Verification items for this drawing (mm, ordinates from the low corner). A direction names the side the tool comes from. Round coordinates to 2 decimals unless told otherwise and drop trailing zeros. Order: outer loops, then holes, each group sorted by start corner. A loop starts at its lowest first (then second) coordinate and runs counter-clockwise, first axis right, second up. Notation, with made-up numbers: (73.5, 54.5) -> (129.5, 54.5) arc R31 ccw to (129.5, 84.5) -> close; hole circle Ø1 at (-22.5, -27.75). An arc over 180 degrees is marked (long way). Put each result on its own line as item: value.
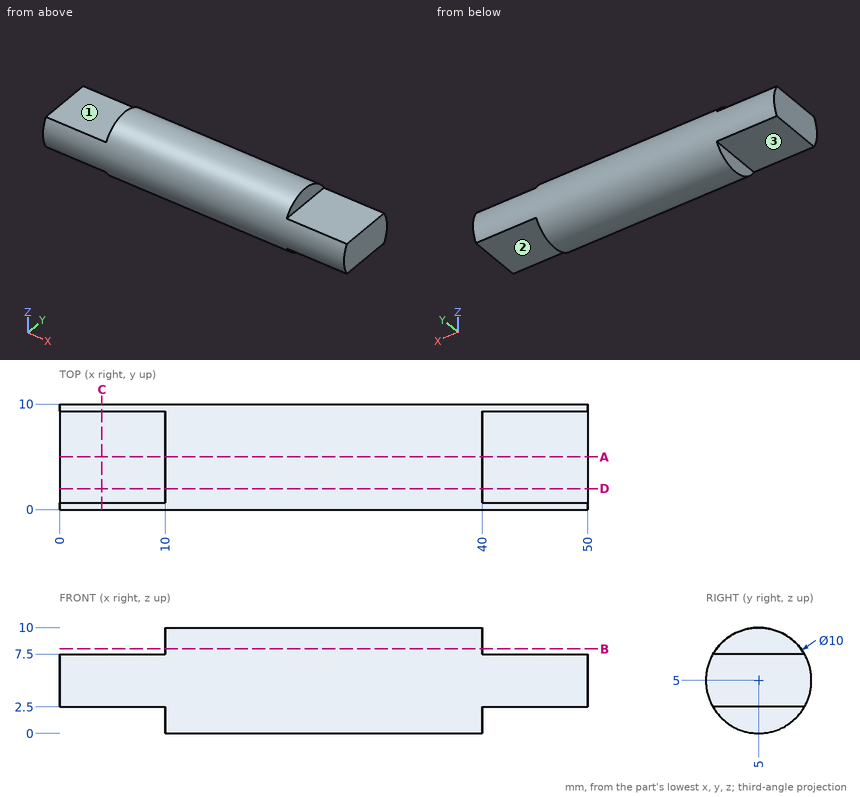
Item 1: Section check B-B on z = 8. Record the boundary of the cut face in (x, y), then the cut area to 3 significant figures.
Check sheet entries:
outline: (10, 1) -> (40, 1) -> (40, 9) -> (10, 9) -> close
area: 240 mm^2
Item 2: Material ranges on L1, parallel to X at y = 1.5, z = 8.5; L2, parallel to Z at x = 6, y = 6.5; L3, parallel to Z at x = 19, y = 4.75, recorded low to high. Write a range as [from, to].
Check sheet entries:
L1: x = [10, 40]
L2: z = [2.5, 7.5]
L3: z = [0.01, 9.99]
Item 3: Section check D-D on y = 2. Record the boundary of the cut face in (x, z), then the cut area to 3 significant figures.
Check sheet entries:
outline: (0, 2.5) -> (10, 2.5) -> (10, 1) -> (40, 1) -> (40, 2.5) -> (50, 2.5) -> (50, 7.5) -> (40, 7.5) -> (40, 9) -> (10, 9) -> (10, 7.5) -> (0, 7.5) -> close
area: 340 mm^2
Item 4: Tool access check on the marked faces 1, 2 and 3. Record the directions out of +Z, -Z, +X, -X, +Y, -Y that give a thin tool (end or side, any length) a straight path to the whole face; none if there is none.
Check sheet entries:
face 1: +Z, -X, +Y, -Y
face 2: -Z, +X, +Y, -Y
face 3: -Z, -X, +Y, -Y
Item 5: Gauge pin test, flat ends, axial feed: pin 1 Ø4 at (x, y) = (35.5, 3.5) entering from +Z; pin 2 Ø1.2 at (y, z) = (6.5, 8.5) entering from -X; pin 3 Ø0.8 at (y, z) = (6.5, 1.5) entering from +X; pin 4 Ø4.5 at (x, y) = (3.5, 4) entering from -Z. Record the tip position at first contact, or that the pin passes through.
Check sheet entries:
pin 1: stops at z = 10
pin 2: stops at x = 10
pin 3: stops at x = 40
pin 4: stops at z = 2.5
Item 6: Section check C-C on x = 4. Record the boundary of the cut face in (y, z).
Check sheet entries:
outline: (0.67, 2.5) -> (9.33, 2.5) arc R5 ccw to (9.33, 7.5) -> (0.67, 7.5) arc R5 ccw to start
Item 7: Section check A-A on y = 5. Record the boundary of the cut face in (x, z), then the cut area to 3 significant figures.
Check sheet entries:
outline: (0, 2.5) -> (10, 2.5) -> (10, 0) -> (40, 0) -> (40, 2.5) -> (50, 2.5) -> (50, 7.5) -> (40, 7.5) -> (40, 10) -> (10, 10) -> (10, 7.5) -> (0, 7.5) -> close
area: 400 mm^2
